Autodesk Inventor part; units mm, degrees
ref_plane "Work Plane1" through (-5.5, 0, 0) normal (0, 0, 1) x (1, 0, 0)
ref_plane "Work Plane2" through (-5.5, 27.494, 0) normal (-0.3947, -0.9188, 0) x (0, 0, 1)
ref_plane "Work Plane3" through (37.205, 87.7645, 25) normal (0, 1, 0) x (1, 0, 0)
sketch "Sketch1" plane through (0, 0, 0) normal (0, 1, 0) x (-1, 0, 0)
  line L0 (-5.5, -37) -> (5.5, -37)
  line L1 (5.5, -37) -> (5.5, 37)
  line L2 (5.5, 37) -> (-5.5, 37)
  line L3 (-5.5, 37) -> (-5.5, -37)
  line L4 (-5.5, -37) -> (5.5, 37) construction
  line L5 (5.5, -37) -> (-5.5, 37) construction
  line L6 (-5.5, -25) -> (5.5, -25)
  line L7 (5.5, -25) -> (5.5, 25)
  line L8 (5.5, 25) -> (-5.5, 25)
  line L9 (-5.5, 25) -> (-5.5, -25)
  line L10 (-5.5, -25) -> (5.5, 25) construction
  line L11 (5.5, -25) -> (-5.5, 25) construction
  circle A0 centre (0, 30) radius 1.5
  circle A1 centre (0, -30) radius 1.5
  point P0 (0, 0)
  point P1 (0, -37)
  dimension "d0" = 74
  dimension "d1" = 11
  dimension "d2" = 11
  dimension "d3" = 50
  dimension "d4" = 3
  dimension "d5" = 7
  dimension "d6" = 3
  dimension "d7" = 7
extrude "Extrusion1" add sketch "Sketch1" along normal blind 10
sketch "Sketch2" plane through (0, 10, 0) normal (0, 1, 0) x (1, 0, 0)
  line L0 (5.5, 37) -> (-5.5, 37)
  line L1 (4.8, 37) -> (14.8, 37)
  line L2 (14.8, 37) -> (14.8, -37)
  line L3 (14.8, -37) -> (4.8, -37)
  line L4 (4.8, -37) -> (4.8, 37)
  line L5 (5.5, -37) -> (5.5, 37)
  point P0 (0, 0)
  dimension "d10" = 74
  dimension "d11" = 0.7
  dimension "d12" = 10
extrude "Extrusion2" add sketch "Sketch2" against normal blind 86
ref_plane "Work Plane1" through (-5.5, 0, 0) normal (0, 0, 1) x (1, 0, 0)
sketch "Sketch3" plane through (-5.5, 0, 0) normal (0, 0, 1) x (1, 0, 0)
  line L0 (20.3, 10) -> (0, 10)
  line L1 (0, 10) -> (0, 27.494)
  line L2 (0, 27.494) -> (0.055, 27.494)
  line L3 (20.3, 10) -> (20.3, -76)
  line L4 (20.3, 10) -> (20.3, -22.405)
  line L5 (20.3, 10) -> (52.705, 10) construction
  line L6 (20.3, -22.405) -> (52.705, 10)
  line L7 (20.3, -22.405) -> (66.1276, -22.405) construction
  line L8 (52.705, 10) -> (52.705, 310)
  line L9 (52.705, 10) -> (352.705, 10) construction
  line L10 (0.055, 27.494) -> (10.055, 27.494) construction
  line L11 (52.705, 101.8003) -> (42.705, 101.8003) construction
  line L12 (42.705, 101.8003) -> (42.705, 219.1463) construction
  line L13 (42.705, 101.8003) -> (160.051, 101.8003) construction
  line L14 (0.055, 27.494) -> (42.705, 126.7645)
  line L15 (42.705, 126.7645) -> (52.705, 126.7645)
  point P0 (5.5, 0)
  dimension "d15" = 17.494
  dimension "d18" = 32.405
  dimension "d19" = 90
  dimension "d20" = 45
  dimension "d22" = 90
  dimension "d23" = 10
  dimension "d25" = 10
  dimension "d27" = 90
  dimension "d79" = 66.75
extrude "Extrusion3" add sketch "Sketch3" along normal mid plane 50
ref_plane "Work Plane2" through (-5.5, 27.494, 0) normal (-0.3947, -0.9188, 0) x (0, 0, 1)
sketch "Sketch4" plane through (-5.5, 0, 25) normal (0, 0, 1) x (1, 0, 0)
  line L0 (0, 0) -> (0, 10) construction
  line L1 (0, 10) -> (0, 23.494) construction
  line L2 (0, 23.494) -> (10, 23.494)
  line L3 (10, 23.494) -> (10, 27.494)
  line L4 (10, 27.494) -> (0, 27.494)
  line L5 (0, 27.494) -> (0, 23.494)
  point P0 (5.5, 0)
  dimension "d31" = 13.494
  dimension "d32" = 10
  dimension "d33" = 4
extrude "Extrusion4" cut sketch "Sketch4" against normal blind 269.75
sketch "Sketch5" plane through (-5.5, 27.494, 0) normal (-0.3947, -0.9188, 0) x (0, 0, 1)
  circle A0 centre (0, 14.9495) radius 25
  line L0 (-25, -0.0505) -> (25, -0.0505)
  point P0 (0, -15.9064)
  dimension "d36" = 50
  dimension "d37" = 15
ref_plane "Work Plane3" through (37.205, 87.7645, 25) normal (0, 1, 0) x (1, 0, 0)
extrude "Extrusion5" cut sketch "Sketch5" along normal blind 54.3375 and the other way blind 67.371
ref_plane "Work Plane5" through (10.2593, -73.9067, 37) normal (-0.9081, 0.4187, 0) x (0, 0, 1)
ref_plane "Work Plane4" through (14.8, -76, 37) normal (-0.9081, 0.4187, 0) x (0, 0, 1)
sketch "Sketch6" plane through (10.2593, -73.9067, 37) normal (-0.9081, 0.4187, 0) x (0, 0, 1)
  line L0 (-74, 0) -> (0, 0)
  circle A0 centre (-37, 54.5) radius 5.5
  circle A1 centre (-37, 54.5) radius 2
  line L1 (-37, -200) -> (-37, 49)
  line L2 (-37, 60) -> (-37, 200)
  circle A2 centre (-47, 30.8) radius 5.5
  circle A3 centre (-47, 30.8) radius 2
  circle A4 centre (-27, 30.8) radius 5.5
  circle A5 centre (-27, 30.8) radius 2
  point P0 (-37, 62.8227)
  point P1 (-37, 0)
  dimension "d43" = 400
  dimension "d44" = 11
  dimension "d45" = 4
  dimension "d46" = 11
  dimension "d47" = 4
  dimension "d48" = 54.5
  dimension "d49" = 23.7
  dimension "d91" = 10
extrude "Extrusion6" cut sketch "Sketch6" along normal blind 15 contours A0 | A1 | A2 | A3 | A4 | A5
extrude "Extrusion7" cut sketch "Sketch6" along normal blind 25.925 contours A0 | A1
extrude "Extrusion8" cut sketch "Sketch6" along normal blind 34.505 contours A1 | A3 | A5
ref_plane "Work Plane6" through (69.3627, 112.9485, -25) normal (-0.9188, 0.3947, 0) x (0, 0, 1)
sketch "Sketch7" plane through (69.3627, 112.9485, -25) normal (-0.9188, 0.3947, 0) x (0, 0, 1)
  line L0 (0, 0) -> (50, 0)
  line L1 (25, 150) -> (25, -150)
  line L2 (25, 150) -> (325, 150) construction
  line L3 (38, 10) -> (12, 10) construction
  line L4 (12, 10) -> (12, -29) construction
  line L5 (12, -29) -> (38, -29) construction
  line L6 (38, -29) -> (38, 10) construction
  circle A0 centre (38, 10) radius 2
  circle A1 centre (38, 10) radius 5
  circle A2 centre (38, -29) radius 2
  circle A3 centre (38, -29) radius 5
  circle A4 centre (12, 10) radius 2
  circle A5 centre (12, 10) radius 5
  circle A6 centre (12, -29) radius 2
  circle A7 centre (12, -29) radius 5
  line L7 (0, 3.9474) -> (50, 3.9474)
  point P0 (25, -131.1566)
  point P1 (25, 0)
  dimension "d57" = 300
  dimension "d58" = 90
  dimension "d63" = 26
  dimension "d64" = 39
  dimension "d67" = 4
  dimension "d68" = 10
  dimension "d69" = 10
  dimension "d70" = 4
  dimension "d78" = 13
  dimension "d85" = 10
fillet "Fillet1" radius 5 2 edges at (14.8, -33, 37) (14.8, -33, -37)
sketch "Sketch8" plane through (-5.5, 0, -25) normal (0, 0, -1) x (-1, 0, 0)
  line L0 (-52.705, 126.7645) -> (-42.705, 126.7645) construction
  line L1 (-42.705, 126.7645) -> (-52.705, 126.7645) construction
  line L2 (-52.705, 10) -> (-52.705, 126.7645)
  line L3 (-0.055, 27.494) -> (-42.705, 126.7645)
  line L4 (-42.705, 126.7645) -> (-52.705, 150.0402)
  line L5 (-52.705, 126.7645) -> (-42.705, 126.7645)
  line L6 (-52.705, 150.0402) -> (-62.705, 150.0402)
  line L7 (-62.705, 150.0402) -> (-52.705, 10)
  point P0 (-5.5, 0)
  dimension "d80" = 66.75
  dimension "d88" = 10
extrude "Extrusion13" add sketch "Sketch8" against normal blind 50
extrude "Extrusion9" cut sketch "Sketch7" along normal blind 28.9375 contours A0 | A1 | A2 | A3 | A4 | A5 | A6 | A7
extrude "Extrusion10" cut sketch "Sketch7" along normal blind 43.9375 contours A0 | A2 | A4 | A6
ref_plane "Work Plane8" through (23.154, -45.9359, -10) normal (0, 0, -1) x (-1, 0, 0)
ref_plane "Work Plane7" through (23.154, -45.9359, -12) normal (0, 0, -1) x (-1, 0, 0)
equation "\"d6\" = d4"
equation "\"d46\" = d44"
equation "\"d47\" = d45"
equation "\"d69\" = d68"
equation "\"d70\" = d67"
equation "\"d78\" = 0.5 * d63"
equation "\"d85\" = screw_offset"
equation "\"screw_offset\" = 10"
properties part number "Camera_Bracket"
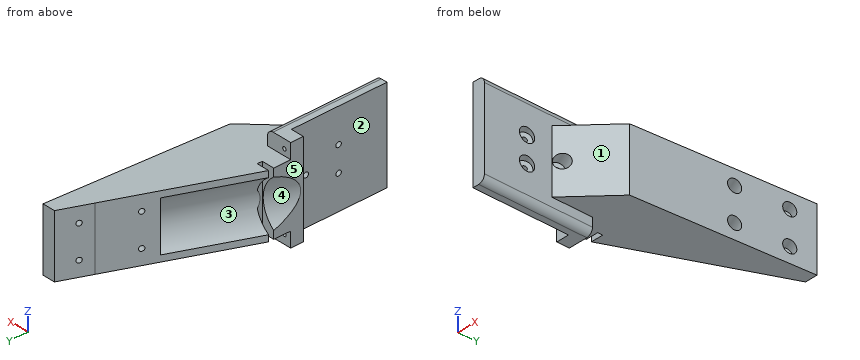
The model under review builds one solid part; all positions refer to its coordinate system, in mm. Face numbers are marked on the shaded views. A direction names the side the tool comes from. Coordinates: 2 decimals unless noted, no trailing zeros. Loops run counter-clockwise (first coordinate to the right, second up) from the corner with the lowest first, then second, coordinate; pieces in that order, holes last. Notation, with made-up numbers: (67, 31.5) -> (119, 31.5) arc R27 ccw to (119, 56.5) -> close; hole circle Ø5 at (25.25, 57.25). An arc over 180 degrees is marked (long way). Use a Markdown table: item, result. Add a question column.
1. To check wall thickness, follow line 1 (Z direction, x = 0, y = 4); line 2 (Z direction, x = 53, y = 129.5); line 3 (Z direction, x = 27, y = 19). State the ranges of each line that lie inside material, in increasing order.
2. Machinability: for the marked faces 1 and 2, which of the approach directions +Z, -Z, +X, -X, +Y, -Y give a long, thin tool a straight path to every point of the face, cutting with its end or side? Answer none if there is none.
3. Clearance check with flat-ended pins moving along their axes: pin 1 Ø3.5 at (x, z) = (4.5, 28) entering from +Y; pin 2 Ø4 at (x, z) = (24, 22) entering from -Y (3 decimals); pin 3 Ø6 at (x, y) = (19, 38.5) entering from -Z. State where each tip first meets the part, or that it passes through.
4. Add section A-A on y = -4.5. Write out the cut boundary in (x, z) (3 decimals).
5. Draft analysis for pull direction Z (two halves, no side actions). For the marked faces 3, 4 and 5, state which applies: pulls with the +Z half, pulls with the -Z half, needs draft (parallel to the pull), parting line crosses it, or undercut.
Returned:
| question | item | result |
|---|---|---|
| 1 | line 1 | z = -37 to -31.5, -28.5 to 28.5, 31.5 to 37 |
| 1 | line 2 | z = -25 to -17.84, -8.16 to 8.16, 17.84 to 25 |
| 1 | line 3 | z = -25 to 25 |
| 2 | face 1 | +Z, -Z, +X, -Y |
| 2 | face 2 | +Z, -Z, -X, -Y |
| 3 | pin 1 | stops at y = 10 |
| 3 | pin 2 | stops at y = -15.205 |
| 3 | pin 3 | stops at z = -25 |
| 4 | outline | (4.8, -37) -> (9.8, -37) arc R5 ccw to (14.8, -32) -> (14.8, -25) -> (32.705, -25) -> (32.705, 25) -> (14.8, 25) -> (14.8, 32) arc R5 ccw to (9.8, 37) -> (4.8, 37) -> close |
| 5 | face 3 | undercut |
| 5 | face 4 | undercut |
| 5 | face 5 | needs draft |
